Here's the drawing with two shaded views (mm, measured from the low corner). I have some questions. Round coordinates to 2 decimals unless told otherwise and drop trailing zeros. Order: outer loops, then holes, each group sorted by start corner. A loop starts at its lowest first (then second) coordinate and runs counter-clockwise, first axis right, second up.
Q1. If we section it at C-C (z = 1.2): Please give me the cut outline in (x, y) (1 decimal).
Q2. If I drill on line 1 (Y direction, x = 50, z = 2.35) (1 decimal); line 2 (X direction, y = 29, z = 0.4) (1 decimal); line 3 (X direction, y = 23.5, z = 0.45) (1 decimal), over which ranges is the centre line in solid material (lowest first)?
Q3. If we section it at D-D (y = 35.5): Please give me the cut outline in (x, z) (1 decimal).
Q4. If we section it at B-B (x = 50): Please give me the cut outline in (y, z) (1 decimal).
Q5. If we section it at A-A (y = 10): Please give me the cut outline in (x, z).
Q6. Will these pins go through, and if not, where does the flat tip stop? P1, Ø1.5, axis at x = 39.5, z = 4, coming from the +Y side; P2, Ø1, axis at x = 15, z = 2, coming from the +Y side (1 decimal); P3, Ø3.5, axis at x = 10, y = 10, coming from the -Z side.
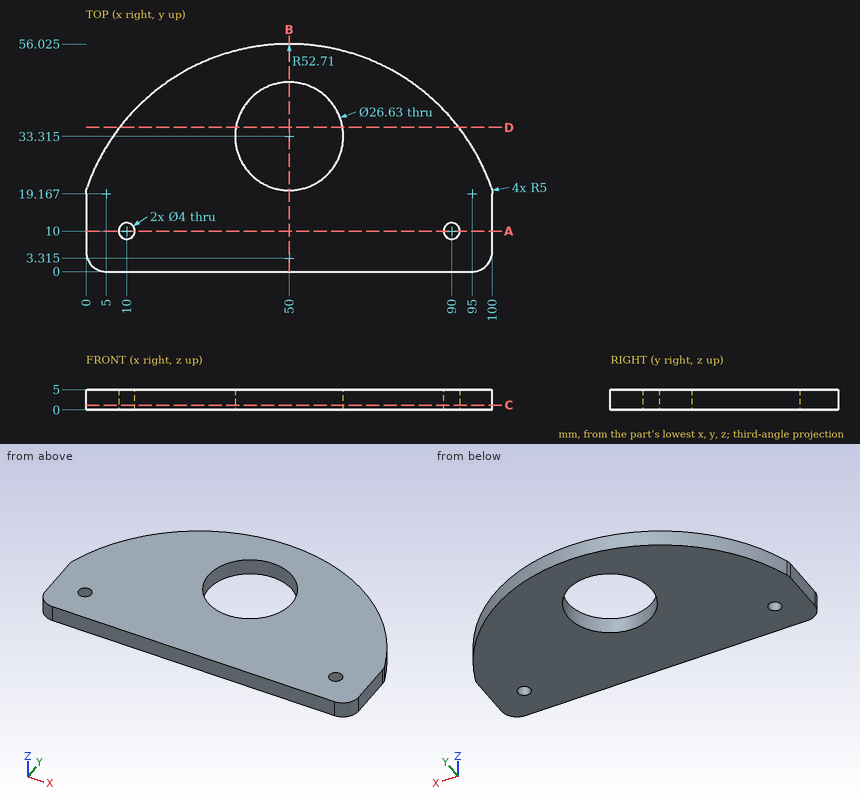
Solution:
1. outline: (0, 5) arc R5 ccw to (5, 0) - (95, 0) arc R5 ccw to (100, 5) - (100, 19.2) arc R5 ccw to (99.7, 20.8) arc R52.7 ccw to (0.3, 20.8) arc R5 ccw to (0, 19.2) - close; hole circle Ø4 at (10, 10); hole circle Ø26.6 at (50, 33.3); hole circle Ø4 at (90, 10)
2. line 1: y = 0 to 20, 46.6 to 56
2. line 2: x = 4 to 37.4, 62.6 to 96
2. line 3: x = 1.3 to 41, 59 to 98.7
3. outline: (8.3, 0) - (36.9, 0) - (36.9, 5) - (8.3, 5) - close; (63.1, 0) - (91.7, 0) - (91.7, 5) - (63.1, 5) - close
4. outline: (0, 0) - (20, 0) - (20, 5) - (0, 5) - close; (46.6, 0) - (56, 0) - (56, 5) - (46.6, 5) - close
5. outline: (0, 0) - (8, 0) - (8, 5) - (0, 5) - close; (12, 0) - (88, 0) - (88, 5) - (12, 5) - close; (92, 0) - (100, 0) - (100, 5) - (92, 5) - close
6. P1: stops at y = 55.12
6. P2: stops at y = 43.2
6. P3: passes through
